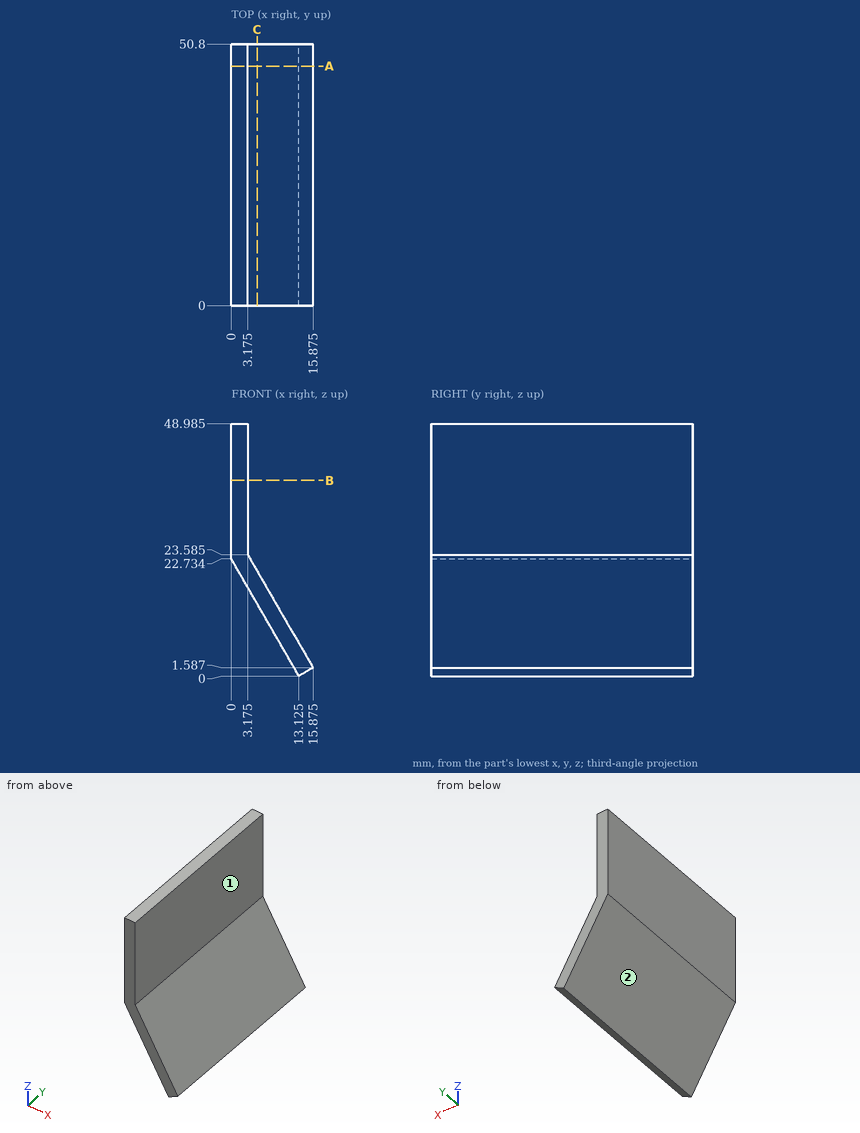
For this review, use the dimensioned drawing (mm, ordinates from the lowest corner) and the shaded views. A direction names the side the tool comes from. Give positions to 0.01 mm unless a question says otherwise; leave off trailing zeros. Order: outer loops, then holes, each group sorted by start corner. A loop starts at its lowest first (then second) coordinate and runs counter-clockwise, first axis right, second up. Notation, with made-up numbers: M -28.75,43.25 L -11.75,43.25 A36 cw -11.75,78.25 Z; hole C 74,-12.5 d10. An arc over 180 degrees is marked long. One line per question, with ' | ' between items. Start each with the question number.
1) Clearance check with flat-ended pins moving along their axes: P1, Ø10, axis at y = 28.5, z = 25.5, coming from the -X side; P2, Ø2, axis at y = 39, z = 7, coming from the +X side; P3, Ø7.5, axis at y = 13, z = 39, coming from the +X side (1 decimal). State where each tip first meets the part, or that it passes through.
2) Consider section B-B, the plane z = 38. Give the boundary of the cut face in (x, y) (1 decimal).
3) For the marked faces 1 and 2, list the 3-axis set-ups (+Z, -Z, +X, -X, +Y, -Y) from which the entire face can be reached by the end or side of a thin tool; tool diameter is ignored.
4) Consider section C-C, the plane x = 5. Give the boundary of the cut face in (y, z).
5) Wall thickness on L1, parallel to X at y = 44.5, z = 38.5 (1 decimal); L2, parallel to Z at x = 15.25, y = 7.5 (1 decimal); L3, parallel to Z at x = 15, y = 45.5 (1 decimal): over which ranges is each line inside the solid? List them lowest first. Write a range as from..to.
6) Consider section A-A, the plane y = 46.5. Give the boundary of the cut face in (x, z) (1 decimal), then the cut area to 3 significant figures.
Found:
1) P1: stops at x = 0 | P2: stops at x = 13.33 | P3: stops at x = 3.2
2) outline: M 0,0 L 3.2,0 L 3.2,50.8 L 0,50.8 Z
3) face 1: +Z, +X, +Y, -Y | face 2: -Z, -X, +Y, -Y
4) outline: M 0,14.07 L 50.8,14.07 L 50.8,20.42 L 0,20.42 Z
5) L1: x = 0..3.2 | L2: z = 1.2..2.7 | L3: z = 1.1..3.1
6) outline: M 0,22.7 L 13.1,0 L 15.9,1.6 L 3.2,23.6 L 3.2,49 L 0,49 Z | area: 164 mm²
